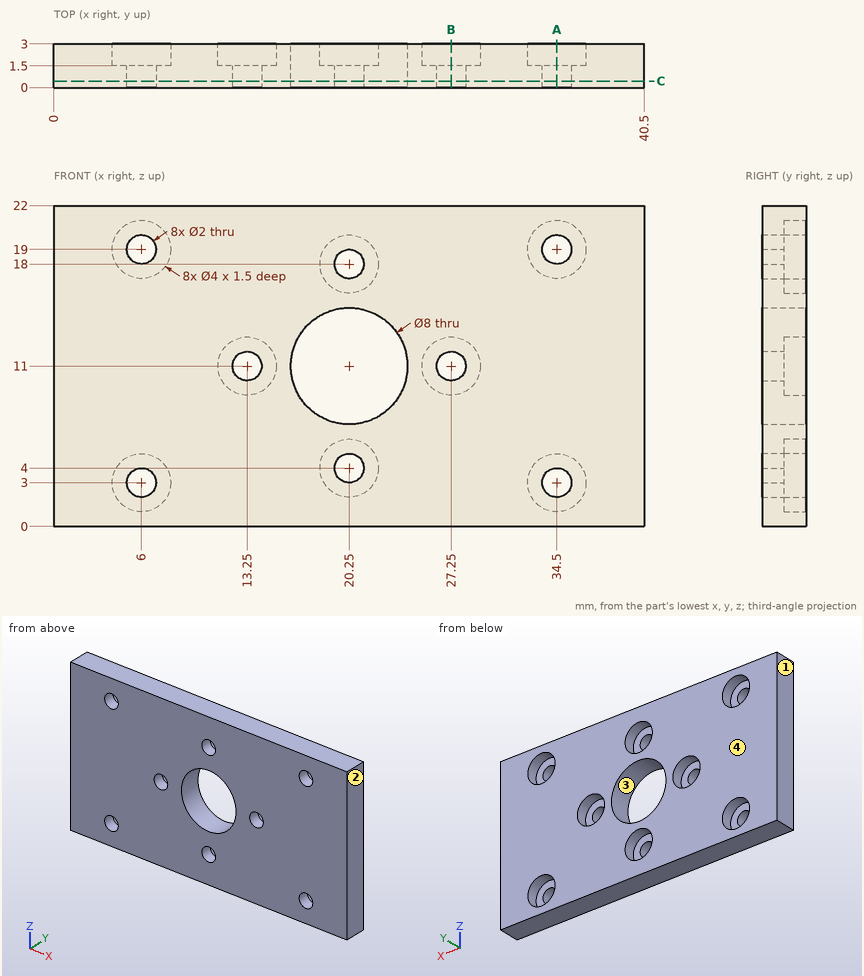
For this review, use the dimensioned drawing (mm, ordinates from the lowest corner) and the shaded views. Coordinates: 2 decimals unless noted, no trailing zeros. Loops run counter-clockwise (first coordinate to the right, second up) from the corner with the lowest first, then second, coordinate; pieces in that order, holes last. Notation, with made-up numbers: (-32, 49.25) -> (-13, 49.25) arc R28 cw to (-13, 69.25) -> close; hole circle Ø8 at (56.25, 45). An arc over 180 degrees is marked (long way). Return JSON: item names as keys, results as strings. Group by question number.
(1) Mouldability with a two-part tool opening along X and no side actions: class the marked faces 1, 2, 3 and 4 as pulls with the +X half, pulls with the -X half, needs draft (parallel to the pull), parting line crosses it, or undercut.
(2) Consider section A-A, the plane x = 34.5. Give the boundary of the cut face in (y, z), plus the area to 3 significant figures.
(3) For pin 1 Ø3 at (x, z) = (6, 3) entering from +Y; pin 2 Ø3 at (x, z) = (35, 18.5) entering from +Y, all flat-tipped, find the tip position at first contact; note any pin that passes through.
(4) Consider section C-C, the plane y = 0.45. Count the separate pieces of the cut face and the enclosed holes in it, plus the area to 3 significant figures.
(5) To check wall thickness, follow L1, parallel to Z at x = 34.5, y = 0.5; L2, parallel to Z at x = 34.5, y = 2.35; L3, parallel to Z at x = 20.25, y = 1.8. State the ranges of each line that lie inside material, in increasing order.
(6) Consider section B-B, the plane x = 27.25. Give the boundary of the cut face in (y, z), plus the area to 3 significant figures.
Results below:
{
 "1": {"face 1": "pulls with the -X half", "face 2": "pulls with the +X half", "face 3": "undercut", "face 4": "needs draft"},
 "2": {"outline": "(0, 0) -> (3, 0) -> (3, 1) -> (1.5, 1) -> (1.5, 2) -> (0, 2) -> close; (0, 4) -> (1.5, 4) -> (1.5, 5) -> (3, 5) -> (3, 17) -> (1.5, 17) -> (1.5, 18) -> (0, 18) -> close; (0, 20) -> (1.5, 20) -> (1.5, 21) -> (3, 21) -> (3, 22) -> (0, 22) -> close", "area": "48.0 mm2"},
 "3": {"pin 1": "stops at y = 1.5", "pin 2": "stops at y = 3"},
 "4": {"separate pieces": "1", "enclosed holes": "9", "area": "816 mm2"},
 "5": {"L1": "z = 0 to 2, 4 to 18, 20 to 22", "L2": "z = 0 to 1, 5 to 17, 21 to 22", "L3": "z = 0 to 2, 6 to 7, 15 to 16, 20 to 22"},
 "6": {"outline": "(0, 0) -> (3, 0) -> (3, 9) -> (1.5, 9) -> (1.5, 10) -> (0, 10) -> close; (0, 12) -> (1.5, 12) -> (1.5, 13) -> (3, 13) -> (3, 22) -> (0, 22) -> close", "area": "57.0 mm2"}
}
